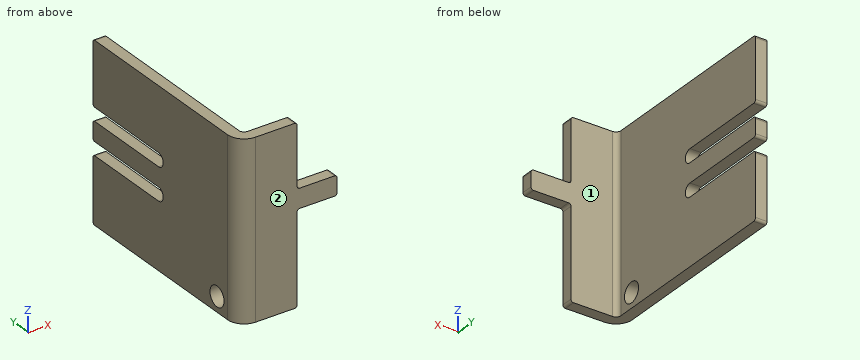
from build123d import *

# Parameters (mm, degrees)
BASE_FLANGE1_DEPTH       = 2.3
SKETCHED_BEND1_OUTLINE_W = 2.3
SKETCHED_BEND1_OUTLINE_H = 35
SKETCHED_BEND1_DEPTH     = 38.388606051
SKETCHED_START           = 38.709564051
SKETCHED_BEND1_2_DEPTH   = 1.979042
SKETCHED_START_2         = 38.388606051
SKETCHED_BEND1_3_DEPTH   = 3.3
SKETCHED_START_3         = -17.5
SKETCHED_BEND1_4_DEPTH   = 35
SKETCH7_R                = 2
CUT_EXTRUDE1_DEPTH       = 10


with BuildPart() as part:
    # Base-Flange1: sheet metal written as solids
    # Sketch1 → Base-Flange1 (new body)
    with BuildSketch(Plane(origin=(0, 0, 0), x_dir=(1, 0, 0), z_dir=(0, 1, 0))):
        with BuildLine():
            Line((0, 17), (0, 4.83))
            ThreePointArc((0, 4.83), (0.146446609, 4.476446609), (0.5, 4.33))
            Line((0.5, 4.33), (18.67, 4.33))
            ThreePointArc((18.67, 4.33), (20, 3), (18.67, 1.67))
            Line((18.67, 1.67), (0.5, 1.67))
            ThreePointArc((0.5, 1.67), (0.146446609, 1.523553391), (0, 1.17))
            Line((0, 1.17), (0, -1.67))
            ThreePointArc((0, -1.67), (0.146446609, -2.023553391), (0.5, -2.17))
            Line((0.5, -2.17), (18.67, -2.17))
            ThreePointArc((18.67, -2.17), (20, -3.5), (18.67, -4.83))
            Line((18.67, -4.83), (0.5, -4.83))
            ThreePointArc((0.5, -4.83), (0.146446609, -4.976446609), (0, -5.33))
            Line((0, -5.33), (0, -17))
            ThreePointArc((0, -17), (0.146446609, -17.353553391), (0.5, -17.5))
            Line((0.5, -17.5), (49.5, -17.5))
            ThreePointArc((49.5, -17.5), (49.853553391, -17.353553391), (50, -17))
            Line((50, -17), (50, -5.42))
            ThreePointArc((50, -5.42), (50.146446609, -5.066446609), (50.5, -4.92))
            Line((50.5, -4.92), (57.5, -4.92))
            ThreePointArc((57.5, -4.92), (57.853553391, -4.773553391), (58, -4.42))
            Line((58, -4.42), (58, -1.58))
            ThreePointArc((58, -1.58), (57.853553391, -1.226446609), (57.5, -1.08))
            Line((57.5, -1.08), (50.5, -1.08))
            ThreePointArc((50.5, -1.08), (50.146446609, -0.933553391), (50, -0.58))
            Line((50, -0.58), (50, 17))
            ThreePointArc((50, 17), (49.853553391, 17.353553391), (49.5, 17.5))
            Line((49.5, 17.5), (0.5, 17.5))
            ThreePointArc((0.5, 17.5), (0.146446609, 17.353553391), (0, 17))
        make_face()
    extrude(amount=-BASE_FLANGE1_DEPTH)

    # Sketched Bend1: read off the stored shape, not the designer's step
    # Sketched Bend1 outline → Sketched Bend1 (cut)
    with BuildSketch(Plane.YZ):
        with Locations((-1.15, 0)):
            Rectangle(SKETCHED_BEND1_OUTLINE_W, SKETCHED_BEND1_OUTLINE_H)
    extrude(amount=SKETCHED_BEND1_DEPTH, mode=Mode.SUBTRACT)

    # Sketched Bend1 2 outline → Sketched Bend1 2 (add)
    with BuildSketch(Plane.YZ.offset(SKETCHED_START)):
        with BuildLine():
            Line((0, -17.5), (38.811393949, -17.5))
            ThreePointArc((38.811393949, -17.5), (39.164947339, -17.353553391), (39.311393949, -17))
            Line((39.311393949, -17), (39.311393949, -4.83))
            ThreePointArc((39.311393949, -4.83), (39.16494734, -4.476446609), (38.811393949, -4.33))
            Line((38.811393949, -4.33), (20.641393949, -4.33))
            ThreePointArc((20.641393949, -4.33), (19.311393949, -3), (20.641393949, -1.67))
            Line((20.641393949, -1.67), (38.811393949, -1.67))
            ThreePointArc((38.811393949, -1.67), (39.16494734, -1.523553391), (39.311393949, -1.17))
            Line((39.311393949, -1.17), (39.311393949, 1.67))
            ThreePointArc((39.311393949, 1.67), (39.16494734, 2.023553391), (38.811393949, 2.17))
            Line((38.811393949, 2.17), (20.641393949, 2.17))
            ThreePointArc((20.641393949, 2.17), (19.311393949, 3.5), (20.641393949, 4.83))
            Line((20.641393949, 4.83), (38.811393949, 4.83))
            ThreePointArc((38.811393949, 4.83), (39.16494734, 4.976446609), (39.311393949, 5.33))
            Line((39.311393949, 5.33), (39.311393949, 17))
            ThreePointArc((39.311393949, 17), (39.164947339, 17.353553391), (38.811393949, 17.5))
            Line((38.811393949, 17.5), (0, 17.5))
            Line((0, 17.5), (0, -17.5))
        make_face()
    extrude(amount=SKETCHED_BEND1_2_DEPTH)

    # Sketched Bend1 3 outline → Sketched Bend1 3 (add)
    with BuildSketch(Plane.YZ.offset(SKETCHED_START_2)):
        with BuildLine():
            Line((0, -17.5), (38.811393949, -17.5))
            ThreePointArc((38.811393949, -17.5), (39.164947339, -17.353553391), (39.311393949, -17))
            Line((39.311393949, -17), (39.311393949, -4.83))
            ThreePointArc((39.311393949, -4.83), (39.16494734, -4.476446609), (38.811393949, -4.33))
            Line((38.811393949, -4.33), (20.641393949, -4.33))
            ThreePointArc((20.641393949, -4.33), (19.311393949, -3), (20.641393949, -1.67))
            Line((20.641393949, -1.67), (38.811393949, -1.67))
            ThreePointArc((38.811393949, -1.67), (39.16494734, -1.523553391), (39.311393949, -1.17))
            Line((39.311393949, -1.17), (39.311393949, 1.67))
            ThreePointArc((39.311393949, 1.67), (39.16494734, 2.023553391), (38.811393949, 2.17))
            Line((38.811393949, 2.17), (20.641393949, 2.17))
            ThreePointArc((20.641393949, 2.17), (19.311393949, 3.5), (20.641393949, 4.83))
            Line((20.641393949, 4.83), (38.811393949, 4.83))
            ThreePointArc((38.811393949, 4.83), (39.16494734, 4.976446609), (39.311393949, 5.33))
            Line((39.311393949, 5.33), (39.311393949, 17))
            ThreePointArc((39.311393949, 17), (39.164947339, 17.353553391), (38.811393949, 17.5))
            Line((38.811393949, 17.5), (0, 17.5))
            Line((0, 17.5), (0, -17.5))
        make_face()
    extrude(amount=SKETCHED_BEND1_3_DEPTH)

    # Sketched Bend1 4 outline → Sketched Bend1 4 (cut)
    with BuildSketch(Plane.XY.offset(SKETCHED_START_3)):
        with BuildLine():
            Line((41.688606051, 39.311393949), (40.688606051, 39.311393949))
            Line((40.688606051, 39.311393949), (40.688606051, 1))
            ThreePointArc((40.688606051, 1), (40.98149927, 0.292893219), (41.688606051, 0))
            Line((41.688606051, 0), (41.688606051, 39.311393949))
        make_face()
        with BuildLine():
            ThreePointArc((41.688606051, -2.3), (39.355153673, -1.333452378), (38.388606051, 1))
            Line((38.388606051, 1), (38.388606051, -2.3))
            Line((38.388606051, -2.3), (41.688606051, -2.3))
        make_face()
    extrude(amount=SKETCHED_BEND1_4_DEPTH, mode=Mode.SUBTRACT)

    # Sketch7 → Cut-Extrude1 (cut)
    with BuildSketch(Plane.ZY.offset(-38.388606051)):
        with Locations(Location((-14.5, 4, 0), (0, 0, 270))):
            Circle(SKETCH7_R)
    extrude(amount=-CUT_EXTRUDE1_DEPTH, mode=Mode.SUBTRACT)


solid = part.part
Check sheet for the modelled part. Datum: model origin and axes. Units: mm. Face numbers are marked on the shaded views. A direction names the side the tool comes from. Coordinates: 2 decimals unless noted, no trailing zeros. Write each loop counter-clockwise with the first axis right and the second up, starting at its lowest first coordinate (ties: lowest second). Pieces come first, ordered by that corner, then holes.
Item 1: Scan lines: probe 1 along Z at (x, y) = (40.05, 4); probe 2 along X at (y, z) = (30.5, -4.5); probe 3 along Y at (x, z) = (41.75, -2.5). Record each from-to range of solid material in increasing order.
Numbers:
probe 1: z = -17.5 to -16.5, -12.5 to 17.5
probe 2: x = 38.39 to 40.69
probe 3: y = -2.3 to 0
Item 2: Cross-section at B-B on y = 34.5. Record the boundary of the cut face in (x, z).
Numbers:
outline: (38.39, -17.5) - (40.69, -17.5) - (40.69, -4.33) - (38.39, -4.33) - close; (38.39, -1.67) - (40.69, -1.67) - (40.69, 2.17) - (38.39, 2.17) - close; (38.39, 4.83) - (40.69, 4.83) - (40.69, 17.5) - (38.39, 17.5) - close
Item 3: Access from +Z, -Z, +X, -X, +Y, -Y to the whole of each face (thin tool, end or side, straight path). Record for the marked faces 1 and 2.
Numbers:
face 1: +Z, -Z, +X, +Y
face 2: +Z, -Z, +X, -X, -Y
Item 4: Cross-section at D-D on x = 43.75. Record the boundary of the cut face in (y, z), then the cut area to 3 significant figures.
Numbers:
outline: (-2.3, -17.5) - (0, -17.5) - (0, 17.5) - (-2.3, 17.5) - close
area: 80.5 mm2
Item 5: Cross-section at A-A on y = 4. Record the boundary of the cut face in (x, z), then the cut area to 3 significant figures.
Numbers:
outline: (38.39, -17.5) - (40.69, -17.5) - (40.69, -16.5) - (38.39, -16.5) - close; (38.39, -12.5) - (40.69, -12.5) - (40.69, 17.5) - (38.39, 17.5) - close
area: 71.3 mm2
Item 6: Depth check by flat-ended pin: pin 1 Ø8 at (y, z) = (28.5, -5.5) entering from +X; pin 2 Ø2.5 at (x, y) = (54.5, -1) entering from +Z; pin 3 Ø0.7 at (y, z) = (-1, -4.5) entering from +X; pin 4 Ø3.5 at (y, z) = (4, -14.5) entering from +X. Enter the tip coordinate at first touch or a pass-through.
Numbers:
pin 1: stops at x = 40.69
pin 2: stops at z = 4.92
pin 3: stops at x = 50
pin 4: passes through
Item 7: Cross-section at C-C on z = -3. Record the boundary of the cut face in (x, y).
Numbers:
outline: (38.39, 1) arc R3.3 ccw to (41.69, -2.3) - (50, -2.3) - (50, 0) - (41.69, 0) arc R1 cw to (40.69, 1) - (40.69, 19.31) - (38.39, 19.31) - close
